```python
from build123d import *

# Parameters (mm, degrees)
F0_W     = 23
F0_H     = 12
F1_DEPTH = 15
F0_W_2   = 5
F0_H_2   = 17.782256
F2_DEPTH = 3


with BuildPart() as f1:
    # F0 (on Front) → F1 (new body)
    with BuildSketch(Plane.XZ):
        Polygon((12.80545, 46.678425), (-16.19455, 46.678425), (-16.19455, 28.896169), (-16.19455, 28.678425), (12.80545, 28.678425), align=None)
        with Locations((-1.62795, 37.678425)):
            Rectangle(F0_W, F0_H, mode=Mode.SUBTRACT)
    extrude(amount=F1_DEPTH)

    # F0 (on Front) → F2 (join)
    with BuildSketch(Plane.XZ):
        with Locations((-18.69455, 37.787297)):
            Rectangle(F0_W_2, F0_H_2)
        Polygon((17.80545, 46.678425), (12.80545, 46.678425), (12.80545, 28.678425), (12.80545, 28.578629), (17.80545, 28.578629), align=None)
    extrude(amount=F2_DEPTH)


solid = f1.part
```
Input: part model. Units: mm. Frame: model coordinates. A direction names the side the tool comes from. Give positions to 0.01 mm unless a question says otherwise; leave off trailing zeros. Write each loop counter-clockwise with the first axis right and the second up, starting at its lowest first coordinate (ties: lowest second). Pieces come first, ordered by that corner, then holes. Notation, with made-up numbers: (1, 52) - (11, 52) arc R26 cw to (11, 91) - close; hole circle Ø1 at (64, 42). An arc over 180 degrees is marked (long way). Write item = value, one per line. Start each with the question number.
1. Section query B-B, the plane z = 42. Output: boundary loops of the cut face in (x, y), then the cut area to 3 significant figures.
2. Ray query, L1, parallel to X at y = -1.25, z = 34.25; L2, parallel to X at y = -12.5, z = 37.75; L3, parallel to Z at x = 7, y = -2.5. Return the intervals inside material, ascending.
3. Mould query, pull axis X, two halves, no side actions, for faces 6 (the flat face through (-21.195, -1, 38)), 7 (the flat face through (-2, -7, 28.678)), 8 (the flat face through (12.805, -9, 38)), 9 (the flat face through (-2, -7, 31.678)). Classes: released by +X, released by -X, zero draft, split by the parting line, or undercut.
4. Access query for faces 1 (the flat face through (15, -3, 38)), 2 (the flat face through (-19, -3, 38)), 3 (the flat face through (9.872, -7, 38)), 4 (the flat face through (-19, -1, 28.896)), 5 (the flat face through (-2, -7, 46.678)). Directions: +Z, -Z, +X, -X, +Y, -Y. A direction counts if a zero-diameter tool reaches every point of the face in a straight line with its end or side. Return the directions, or none.
5. Section query D-D, the plane z = 44.75. Output: boundary loops of the cut face in (x, y).
6. First-contact query: pin 1 Ø1.5 at (x, z) = (15, 39.5) entering from -Y; pin 2 Ø3 at (y, z) = (-11, 41) entering from -X; pin 3 Ø6 at (y, z) = (-8, 38.5) entering from +X. Flat tips, straight axial feed; report the tip coordinate or a pass-through.
7. Section query A-A, the plane y = -7. Output: boundary loops of the cut face in (x, z), then the cut area to 3 significant figures.
8. Section query C-C, the plane x = -0.5. Output: boundary loops of the cut face in (y, z), then the cut area to 3 significant figures.
Check sheet entries:
q1.outline = (-21.19, -3) - (-16.19, -3) - (-16.19, -15) - (-13.13, -15) - (-13.13, 0) - (-21.19, 0) - close; (9.87, -15) - (12.81, -15) - (12.81, -3) - (17.81, -3) - (17.81, 0) - (9.87, 0) - close
q1.area = 120 mm2
q2.L1 = -21.19 to -13.13, 9.87 to 17.81
q2.L2 = -16.19 to -13.13, 9.87 to 12.81
q2.L3 = 28.68 to 31.68, 43.68 to 46.68
q3.face_6 = released by -X
q3.face_7 = zero draft
q3.face_8 = released by +X
q3.face_9 = undercut
q4.face_1 = +Z, -Z, +X, -Y
q4.face_2 = +Z, -Z, -X, -Y
q4.face_3 = +Y, -Y
q4.face_4 = -Z, -X, +Y, -Y
q4.face_5 = +Z, +X, -X, +Y, -Y
q5.outline = (-21.19, -3) - (-16.19, -3) - (-16.19, -15) - (12.81, -15) - (12.81, -3) - (17.81, -3) - (17.81, 0) - (-21.19, 0) - close
q6.pin_1 = -3
q6.pin_2 = -16.19
q6.pin_3 = 12.81
q7.outline = (-16.19, 28.68) - (12.81, 28.68) - (12.81, 46.68) - (-16.19, 46.68) - close; hole (-13.13, 31.68) - (9.87, 31.68) - (9.87, 43.68) - (-13.13, 43.68) - close
q7.area = 246 mm2
q8.outline = (-15, 28.68) - (0, 28.68) - (0, 31.68) - (-15, 31.68) - close; (-15, 43.68) - (0, 43.68) - (0, 46.68) - (-15, 46.68) - close
q8.area = 90.0 mm2
